from build123d import *

# Parameters (mm, degrees)
SKETCH1_W           = 150
SKETCH1_H           = 3
BOSS_EXTRUDE1_DEPTH = 170
SKETCH2_W           = 150
SKETCH2_H           = 5
BOSS_EXTRUDE2_DEPTH = 10
SKETCH3_W           = 100
SKETCH3_H           = 3
BOSS_EXTRUDE3_DEPTH = 3
SKETCH4_W           = 100
SKETCH4_H           = 3
BOSS_EXTRUDE4_DEPTH = 5
SKETCH5_R           = 1.5
CUT_EXTRUDE1_DEPTH  = 191.741316971
SKETCH6_W           = 8
SKETCH6_H           = 10
BOSS_EXTRUDE5_DEPTH = 5
SKETCH8_W           = 8
SKETCH8_H           = 10
BOSS_EXTRUDE6_DEPTH = 5
SKETCH9_R           = 1.5
CUT_EXTRUDE2_DEPTH  = 228.007158477
SKETCH10_W          = 100
SKETCH10_H          = 5
CUT_EXTRUDE3_DEPTH  = 1


with BuildPart() as part:
    # Sketch1 → Boss-Extrude1 (new body)
    with BuildSketch(Plane(origin=(0, 0, 0), x_dir=(1, 0, 0), z_dir=(0, 1, 0))):
        Rectangle(SKETCH1_W, SKETCH1_H)
    extrude(amount=BOSS_EXTRUDE1_DEPTH)

    # Sketch2 → Boss-Extrude2 (add)
    with BuildSketch(Plane(origin=(0, 0, -1.5), x_dir=(-1, 0, 0), z_dir=(0, 0, -1))):
        with Locations((0, 167.5)):
            Rectangle(SKETCH2_W, SKETCH2_H)
    extrude(amount=BOSS_EXTRUDE2_DEPTH)

    # Sketch3 → Boss-Extrude3 (add)
    with BuildSketch(Plane(origin=(0, 0, -1.5), x_dir=(-1, 0, 0), z_dir=(0, 0, -1))):
        with Locations((0, 1.5)):
            Rectangle(SKETCH3_W, SKETCH3_H)
    extrude(amount=BOSS_EXTRUDE3_DEPTH)

    # Sketch4 → Boss-Extrude4 (add)
    with BuildSketch(Plane.XZ):
        with Locations((0, -3)):
            Rectangle(SKETCH4_W, SKETCH4_H)
    extrude(amount=BOSS_EXTRUDE4_DEPTH)

    # Sketch5 → Cut-Extrude1 (cut, through all)
    with BuildSketch(Plane(origin=(0, 170, 0), x_dir=(1, 0, 0), z_dir=(0, 1, 0))):
        with Locations(Location((69, 4.5, 0), (0, 0, 270))):
            Circle(SKETCH5_R)
        with Locations(Location((-69, 4.5, 0), (0, 0, 270))):
            Circle(SKETCH5_R)
    extrude(amount=-CUT_EXTRUDE1_DEPTH, mode=Mode.SUBTRACT)

    # Sketch6 → Boss-Extrude5 (add)
    with BuildSketch(Plane(origin=(75, 0, 0), x_dir=(0, 0, -1), z_dir=(1, 0, 0))):
        with Locations((2.5, 82.5)):
            Rectangle(SKETCH6_W, SKETCH6_H)
    extrude(amount=-BOSS_EXTRUDE5_DEPTH)

    # Sketch8 → Boss-Extrude6 (add)
    with BuildSketch(Plane.ZY.offset(75)):
        with Locations((-2.5, 82.5)):
            Rectangle(SKETCH8_W, SKETCH8_H)
    extrude(amount=-BOSS_EXTRUDE6_DEPTH)

    # Sketch9 → Cut-Extrude2 (cut, through all)
    with BuildSketch(Plane.ZY.offset(75)):
        with Locations((-4, 82.5)):
            Circle(SKETCH9_R)
    extrude(amount=-CUT_EXTRUDE2_DEPTH, mode=Mode.SUBTRACT)

    # Sketch10 → Cut-Extrude3 (cut)
    with BuildSketch(Plane.XY.offset(-1.5)):
        with Locations((0, -2.5)):
            Rectangle(SKETCH10_W, SKETCH10_H)
    extrude(amount=-CUT_EXTRUDE3_DEPTH, mode=Mode.SUBTRACT)


solid = part.part
Geometry: final body of the model. Coordinates: model frame, mm. A direction names the side the tool comes from. Give positions to 0.01 mm unless a question says otherwise; leave off trailing zeros. Write each loop counter-clockwise with the first axis right and the second up, starting at its lowest first coordinate (ties: lowest second). Pieces come first, ordered by that corner, then holes.
(1) First-contact query: P1, Ø4, axis at x = -40.5, y = 41, coming from the -Z side; P2, Ø1.5, axis at x = -72.5, y = 85, coming from the -Z side; P3, Ø2.5, axis at x = -69, z = -4.5, coming from the +Y side. Flat tips, straight axial feed; report the tip coordinate or a pass-through.
(2) Access query for faces 1 (the flat face through (-73, 87.5, -4)), 2 (the flat face through (-70, 84, -5)), 3 (the flat face through (-1, 0, -1)). Directions: +Z, -Z, +X, -X, +Y, -Y. A direction counts if a zero-diameter tool reaches every point of the face in a straight line with its end or side. Return the directions, or none.
(3) Ray query, line 1 (Y direction, x = 71.15, z = -4); line 2 (X direction, y = 167.5, z = -4.5); line 3 (Z direction, x = 71.5, y = 82.5). Return the intervals inside material, ascending.
(4) Cut plane B-B, the plane y = 126.5. Return loops of the section in (x, z).
(5) Cut plane A-A, the plane x = -57. Return loops of the section in (y, z).
(6) Mould query, pull axis Y, two halves, no side actions, for faces 4 (the flat face through (-73, 82, -6.5)), 5 (the flat face through (1, 170, -5)), 6 (the flat face through (73, 87.5, -4)). Classes: released by +Y, released by -Y, zero draft, split by the parting line, or undercut.
Values follow:
1. P1: stops at z = -1.5
1. P2: stops at z = -6.5
1. P3: stops at y = 87.5
2. face 1: -Z, +X, -X
2. face 2: -Z, -Y
2. face 3: +Z, +X, -X, -Y
3. line 1: y = 77.5 to 81, 84 to 87.5, 165 to 170
3. line 2: x = -75 to -70.5, -67.5 to 67.5, 70.5 to 75
3. line 3: z = -6.5 to -5.5, -2.5 to 1.5
4. outline: (-75, -1.5) - (75, -1.5) - (75, 1.5) - (-75, 1.5) - close
5. outline: (0, -1.5) - (165, -1.5) - (165, -11.5) - (170, -11.5) - (170, 1.5) - (0, 1.5) - close
6. face 4: zero draft
6. face 5: released by +Y
6. face 6: undercut
